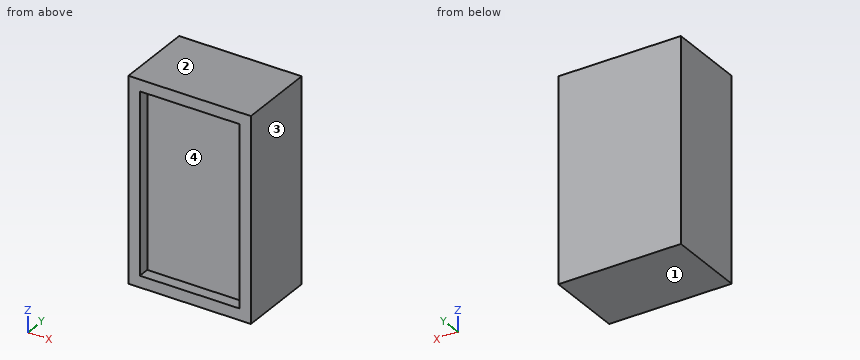
```python
from build123d import *

# Parameters (mm, degrees)
SKETCH1_W           = 320.53572501
SKETCH1_H           = 205.006558649
BOSS_EXTRUDE1_DEPTH = 530
SKETCH2_W           = 260.54
SKETCH2_H           = 470
CUT_EXTRUDE1_DEPTH  = 30


with BuildPart() as part:
    # Sketch1 → Boss-Extrude1 (new body)
    with BuildSketch(Plane.XY.offset(30)):
        with Locations((0, -2.496720675)):
            Rectangle(SKETCH1_W, SKETCH1_H)
    extrude(amount=-BOSS_EXTRUDE1_DEPTH)

    # Sketch2 → Cut-Extrude1 (cut)
    with BuildSketch(Plane.XZ.offset(105)):
        with Locations((0.002137495, -235)):
            Rectangle(SKETCH2_W, SKETCH2_H)
    extrude(amount=-CUT_EXTRUDE1_DEPTH, mode=Mode.SUBTRACT)


solid = part.part
```
Can you work these out from the model? Positions are in its coordinate system, mm. Face numbers are marked on the shaded views. Give positions to 0.01 mm unless a question says otherwise; leave off trailing zeros. Write each loop counter-clockwise with the first axis right and the second up, starting at its lowest first coordinate (ties: lowest second). Pieces come first, ordered by that corner, then holes. Notation, with made-up numbers: (89, 8.25) - (95, 8.25) arc R22 cw to (95, 29.25) - close; hole circle Ø1 at (67.25, -17). An arc over 180 degrees is marked (long way). Write item = value, one per line. Start each with the question number.
1. For pin 1 (5 mm diameter, centred on x = -108.5, z = -259, fed in from -Y), with a flat end and sliding along its axis, tell me the tip position at first contact or that it passes through.
2. Imagine slicing it at A-A (x = 81). Please give me the cut outline in (y, z), and give its area (3 significant figures).
3. Imagine slicing it at B-B (z = -325). Please give me the cut outline in (x, y), and give its area (3 significant figures).
4. Please list where these lines run through material, in increasing order: line 1 (X direction, y = -82.5, z = -164); line 2 (Z direction, x = 91, y = -88); line 3 (Y direction, x = 23, z = -446).
5. Thinking about a two-plate mould opening in Z: for the marked faces 1, 2, 3 and 4, which applies, released by +Z, released by -Z, zero draft, split by the parting line, or undercut?
Worked answers:
q1.pin_1 = -75
q2.outline = (-105, -500) - (100.01, -500) - (100.01, 30) - (-105, 30) - (-105, 0) - (-75, 0) - (-75, -470) - (-105, -470) - close
q2.area = 94,600 mm2
q3.outline = (-160.27, -105) - (-130.27, -105) - (-130.27, -75) - (130.27, -75) - (130.27, -105) - (160.27, -105) - (160.27, 100.01) - (-160.27, 100.01) - close
q3.area = 57,900 mm2
q4.line_1 = -160.27 to -130.27, 130.27 to 160.27
q4.line_2 = -500 to -470, 0 to 30
q4.line_3 = -75 to 100.01
q5.face_1 = released by -Z
q5.face_2 = released by +Z
q5.face_3 = zero draft
q5.face_4 = undercut
